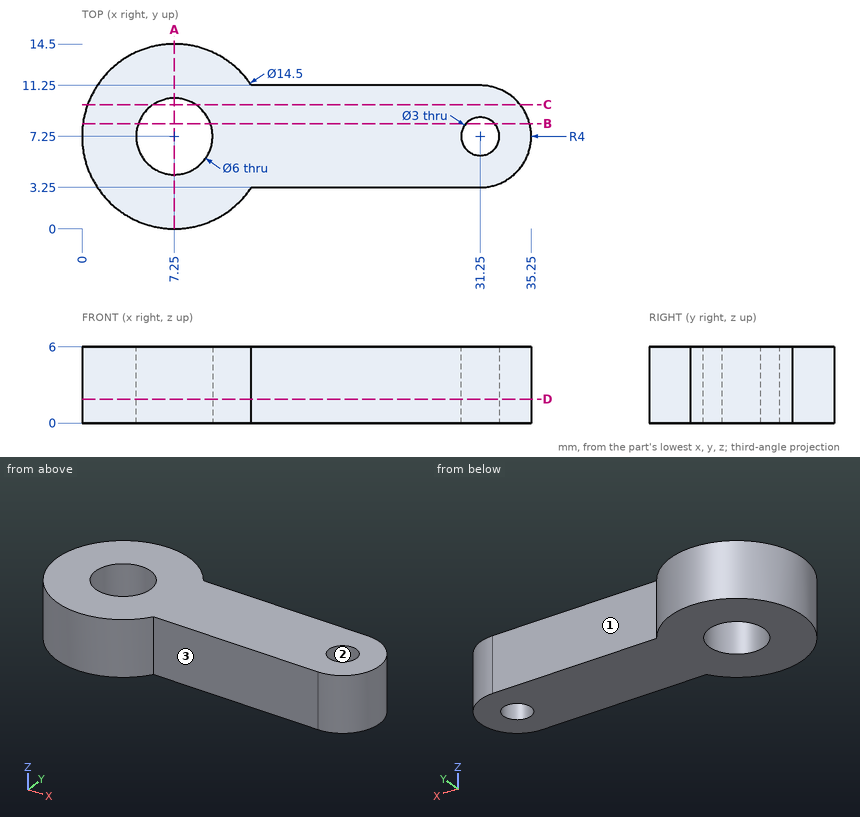
Part print with two shaded views. Sizes in mm from the minimum x, y, z corner. A direction names the side the tool comes from. Round coordinates to 2 decimals unless told otherwise and drop trailing zeros. Loops run counter-clockwise (first coordinate to the right, second up) from the corner with the lowest first, then second, coordinate; pieces in that order, holes last. Notation, with made-up numbers: (31, 0.25) - (71, 0.25) arc R21 cw to (71, 37.25) - close; hole circle Ø11 at (-39.75, -4). An arc over 180 degrees is marked (long way). Answer as a JSON object with one key per item and string values.
Item 1: Band-saw the part on C-C on y = 9.75. List the corners of the cut face in (x, z).
Output:
{"outline": "(0.44, 0) - (5.59, 0) - (5.59, 6) - (0.44, 6) - close; (8.91, 0) - (34.37, 0) - (34.37, 6) - (8.91, 6) - close"}
Item 2: Band-saw the part on B-B on y = 8.25. List the corners of the cut face in (x, z), plus the area to 3 significant figures.
Output:
{"outline": "(0.07, 0) - (4.42, 0) - (4.42, 6) - (0.07, 6) - close; (10.08, 0) - (30.13, 0) - (30.13, 6) - (10.08, 6) - close; (32.37, 0) - (35.12, 0) - (35.12, 6) - (32.37, 6) - close", "area": "163 mm2"}
Item 3: Wall check: L1, parallel to X at y = 8, z = 0.65; L2, parallel to Y at x = 31.25, z = 4.45; L3, parallel to Y at x = 28, z = 4.75. Give the ranges that are in metal, low to high.
Output:
{"L1": "0.04 to 4.35, 10.15 to 29.95, 32.55 to 35.18", "L2": "3.25 to 5.75, 8.75 to 11.25", "L3": "3.25 to 11.25"}
Item 4: Band-saw the part on A-A on x = 7.25. List the corners of the cut face in (y, z), plus the area to 3 significant figures.
Output:
{"outline": "(0, 0) - (4.25, 0) - (4.25, 6) - (0, 6) - close; (10.25, 0) - (14.5, 0) - (14.5, 6) - (10.25, 6) - close", "area": "51.0 mm2"}
Item 5: Tool access for the marked faces 1, 2 and 3: list every direction of +Z, -Z, +X, -X, +Y, -Y with a clear straight run to the whole face (end or side of a thin tool).
Output:
{"face 1": "+Z, -Z, +X, +Y", "face 2": "+Z, -Z", "face 3": "+Z, -Z, +X, -Y"}
Item 6: Pin check, flat tips, straight feed: pin 1 (3 mm diameter, centred on x = 14, y = 3.5, fed in from -Z); pin 2 (3 mm diameter, centred on x = 18.5, z = 1.5, fed in from +Y); pin 3 (3 mm diameter, centred on y = 5, z = 2, fed in from -X); pin 4 (3 mm diameter, centred on y = 10.5, z = 3.5, fed in from +X). Stop position of each tip, or through.
Output:
{"pin 1": "z = 0", "pin 2": "y = 11.25", "pin 3": "x = 0.04", "pin 4": "x = 34.85"}
Item 7: Band-saw the part on D-D on z = 1.9. List the corners of the cut face in (x, y).
Output:
{"outline": "(13.3, 3.25) - (31.25, 3.25) arc R4 ccw to (31.25, 11.25) - (13.3, 11.25) arc R7.25 ccw (long way) to start; hole circle Ø6 at (7.25, 7.25); hole circle Ø3 at (31.25, 7.25)"}
